Here's how the part is built. I have some questions about the finished solid (model axes, mm). Give positions to 0.01 mm unless a question says otherwise; leave off trailing zeros. Loops run counter-clockwise (first coordinate to the right, second up) from the corner with the lowest first, then second, coordinate; pieces in that order, holes last.
Q1. I'm going to push a flat-ended pin straight in: P1, Ø2.5, axis at x = 0, z = 16, coming from the +Y side. Where does the tip first touch, or does it pass through?
Q2. Thinking about a two-plate mould opening in X: for faces 1 (the face through (-10, 0.5, -0.1)), 2 (the face through (5.37, 0.49, -1.19)), 3 (the face through (-0.2, 0.5, -18)), which applies, pulls with the +X half, pulls with the -X half, needs draft (parallel to the pull), parting line crosses it, or undercut?
Q3. Suppose I cut it at B-B (y = 0.3). List the corners of the cut face in (x, z) for me, and give its area (3 significant figures).
Q4. I need wall thicknesses on probe 1 along Z at (x, y) = (0, 0.7); probe 2 along X at (y, z) = (0.45, 2); probe 3 along X at (y, z) = (0.4, 0). Which ranges of each line are inside material? Lowest first, please.
Q5. Suppose I cut it at A-A (z = 16). List the corners of the cut face in (x, y) for me.
Q6. Suppose I cut it at D-D (x = 6). List the corners of the cut face in (y, z) for me, and give its area (3 significant figures).
Q7. Suppose I cut it at C-C (x = -2). List the corners of the cut face in (y, z) for me, and give its area (3 significant figures).
Autodesk Inventor part; units mm, degrees
ref_plane "YZ Plane" through (0, 0, 0) normal (1, 0, 0) x (0, 1, 0)
ref_plane "XZ Plane" through (0, 0, 0) normal (0, 1, 0) x (-1, 0, 0)
ref_plane "XY Plane" through (0, 0, 0) normal (0, 0, 1) x (1, 0, 0)
sketch "Skizze1" plane through (0, 0, 0) normal (0, 1, 0) x (-1, 0, 0)
  line L0 (0, 8) -> (0, -8) construction
  line L1 (-10, 8) -> (-10, -8)
  line L2 (10, -8) -> (10, 8)
  arc A0 (10, 8) -> (-10, 8) centre (0, 8) ccw
  arc A1 (-10, -8) -> (10, -8) centre (0, -8) ccw
  point P0 (0, 0)
  point P1 (0, 0)
  dimension "d0" = 10
  dimension "d1" = 16
extrude "Extrusion1" add sketch "Skizze1" along normal blind 1
sketch "Skizze2" plane through (0, 1, 0) normal (0, 1, 0) x (1, 0, 0)
  point P0 (0, 0)
  point P1 (0, -16)
  point P2 (0, 16)
  dimension "d11" = 32
  dimension "d12" = 16
hole "Bohrung1" at (0, 1, 16) at (0, 1, -16) direction (0, -1, 0) diameter 3.1 depth 1
hole "Bohrung2" at (0, 1, 0) direction (0, -1, 0) diameter 11 depth 1
properties part number "Deckscheibe"
Solutions:
1. P1: passes through
2. face 1: pulls with the -X half
2. face 2: undercut
2. face 3: parting line crosses it
3. outline: (-10, -8) arc R10 ccw to (10, -8) - (10, 8) arc R10 ccw to (-10, 8) - close; hole circle Ø11 at (0, 0); hole circle Ø3.1 at (0, -16); hole circle Ø3.1 at (0, 16)
3. area: 524 mm2
4. probe 1: z = -18 to -17.55, -14.45 to -5.5, 5.5 to 14.45, 17.55 to 18
4. probe 2: x = -10 to -5.12, 5.12 to 10
4. probe 3: x = -10 to -5.5, 5.5 to 10
5. outline: (-6, 0) - (-1.55, 0) - (-1.55, 1) - (-6, 1) - close; (1.55, 0) - (6, 0) - (6, 1) - (1.55, 1) - close
6. outline: (0, -16) - (1, -16) - (1, 16) - (0, 16) - close
6. area: 32.0 mm2
7. outline: (0, -17.8) - (1, -17.8) - (1, -5.12) - (0, -5.12) - close; (0, 5.12) - (1, 5.12) - (1, 17.8) - (0, 17.8) - close
7. area: 25.3 mm2
